Check sheet for the drawn part. Datum: minimum x, y, z corner. Units: mm. A direction names the side the tool comes from. Give positions to 0.01 mm unless a question says otherwise; leave off trailing zeros. Loops run counter-clockwise (first coordinate to the right, second up) from the corner with the lowest first, then second, coordinate; pieces in that order, holes last. Notation, with made-up numbers: (7, 64.25) - (57, 64.25) arc R33 ccw to (57, 98.25) - close; hole circle Ø3 at (64, 58.5). An arc over 180 degrees is marked (long way). Answer in a Markdown table with one row per item.
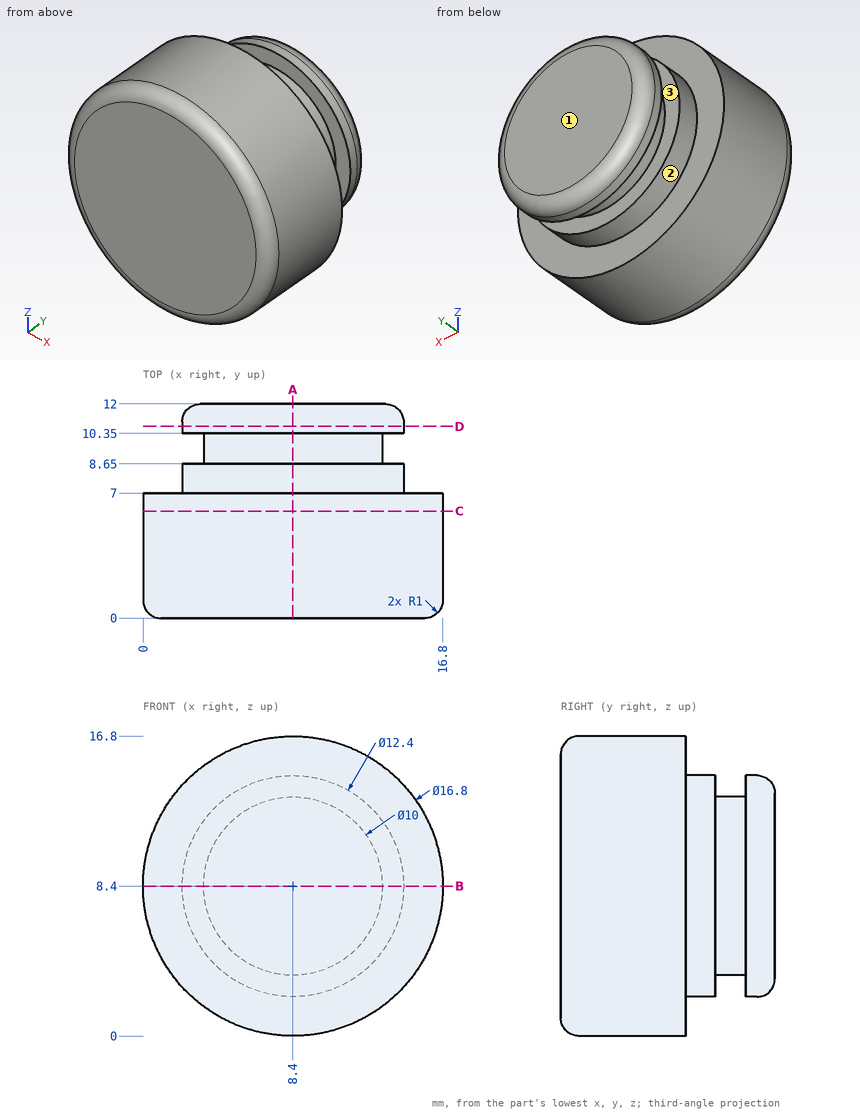
Q1. Sectioned sample at A-A (x = 8.4). Record the cut outline in (y, z), and give its area (3 significant figures).
Completed:
| item | result |
|---|---|
| outline | (0, 1) arc R1 ccw to (1, 0) - (7, 0) - (7, 2.2) - (8.65, 2.2) - (8.65, 3.4) - (10.35, 3.4) - (10.35, 2.2) - (11, 2.2) arc R1 ccw to (12, 3.2) - (12, 13.6) arc R1 ccw to (11, 14.6) - (10.35, 14.6) - (10.35, 13.4) - (8.65, 13.4) - (8.65, 14.6) - (7, 14.6) - (7, 16.8) - (1, 16.8) arc R1 ccw to (0, 15.8) - close |
| area | 175 mm^2 |
Q2. Sectioned sample at B-B (z = 8.4). Record the cut outline in (x, y), and give its area (3 significant figures).
Completed:
| item | result |
|---|---|
| outline | (0, 1) arc R1 ccw to (1, 0) - (15.8, 0) arc R1 ccw to (16.8, 1) - (16.8, 7) - (14.6, 7) - (14.6, 8.65) - (13.4, 8.65) - (13.4, 10.35) - (14.6, 10.35) - (14.6, 11) arc R1 ccw to (13.6, 12) - (3.2, 12) arc R1 ccw to (2.2, 11) - (2.2, 10.35) - (3.4, 10.35) - (3.4, 8.65) - (2.2, 8.65) - (2.2, 7) - (0, 7) - close |
| area | 175 mm^2 |
Q3. Tool access check on the marked faces 1, 2 and 3. Record the directions out of +Z, -Z, +X, -X, +Y, -Y that give a thin tool (end or side, any length) a straight path to the whole face; none if there is none.
Completed:
| item | result |
|---|---|
| face 1 | +Z, -Z, +X, -X, +Y |
| face 2 | +Y |
| face 3 | none |
Q4. Go/stop test with flat-tipped pins: P1, Ø2, axis at x = 3.5, y = 6, coming from the +Z side; P2, Ø3, axis at y = 3, z = 11.5, coming from the +X side; P3, Ø4, axis at x = 15, y = 7.5, coming from the -Z side. Record where each tip stops, or that it passes through.
Completed:
| item | result |
|---|---|
| P1 | z = 15.84 |
| P2 | x = 16.65 |
| P3 | z = 1.41 |
Q5. Thickness scan on line 1 (Y direction, x = 3.25, z = 8.25); line 2 (Y direction, x = 14, z = 5.5); line 3 (X direction, y = 2, z = 8.5). Record the ranges inside material, lowest first.
Completed:
| item | result |
|---|---|
| line 1 | 0 to 8.65, 10.35 to 12 |
| line 2 | 0 to 7 |
| line 3 | 0 to 16.8 |
Q6. Sectioned sample at D-D (y = 10.75). Record the cut outline in (x, z), and give its area (3 significant figures).
Completed:
| item | result |
|---|---|
| outline | circle Ø12.4 at (8.4, 8.4) |
| area | 121 mm^2 |
Q7. Sectioned sample at C-C (y = 6). Record the cut outline in (x, z).
Completed:
| item | result |
|---|---|
| outline | circle Ø16.8 at (8.4, 8.4) |
